Autodesk Inventor part; units mm, degrees
ref_plane "YZ Plane" through (0, 0, 0) normal (1, 0, 0) x (0, 1, 0)
ref_plane "XZ Plane" through (0, 0, 0) normal (0, 1, 0) x (-1, 0, 0)
ref_plane "XY Plane" through (0, 0, 0) normal (0, 0, 1) x (1, 0, 0)
sketch "Sketch1" plane through (0, 0, 0) normal (0, 1, 0) x (-1, 0, 0)
  line L0 (-14.4018, 8.0518) -> (14.4018, 8.0518)
  line L1 (14.4018, 8.0518) -> (14.4018, -8.0518)
  line L2 (14.4018, -8.0518) -> (-14.4018, -8.0518)
  line L3 (-14.4018, -8.0518) -> (-14.4018, 8.0518)
  line L4 (-14.4018, 8.0518) -> (14.4018, -8.0518) construction
  line L5 (14.4018, 8.0518) -> (-14.4018, -8.0518) construction
  point P0 (0, 0)
  dimension "d0" = 28.8036
  dimension "d1" = 16.1036
extrude "Extrusion1" add sketch "Sketch1" along normal blind 17.018
sketch "Sketch2" plane through (0, 17.018, 0) normal (0, 1, 0) x (1, 0, 0)
  circle A0 centre (0, 0) radius 5.9531
  dimension "d4" = 11.9062
extrude "Extrusion2" add sketch "Sketch2" along normal blind 11.811
sketch "Sketch3" plane through (0, 28.829, 0) normal (0, 1, 0) x (1, 0, 0)
  circle A0 centre (0, 0) radius 3.175
  dimension "d7" = 6.35
extrude "Extrusion3" add sketch "Sketch3" along normal blind 16.9926
fillet "Fillet1" radius 3.175 1 edges at (-3.175, 45.8216, 0)
sketch "Sketch4" plane through (0, 0, 0) normal (0, -1, 0) x (1, 0, 0)
  line L0 (-14.4018, 8.0518) -> (14.4018, 8.0518)
  line L1 (0, 8.0518) -> (3.175, 8.0518)
  line L2 (3.175, 8.0518) -> (3.175, 7.2644)
  line L3 (3.175, 7.2644) -> (0, 7.2644)
  line L4 (0, 7.2644) -> (0, 8.0518)
  line L5 (0, 8.0518) -> (-3.175, 8.0518)
  line L6 (-3.175, 8.0518) -> (-3.175, 7.2644)
  line L7 (-3.175, 7.2644) -> (0, 7.2644)
  point P0 (0, 0)
  dimension "d11" = 3.175
  dimension "d12" = 0.7874
extrude "Extrusion4" add sketch "Sketch4" along normal blind 10.795
sketch "Sketch5" plane through (0, 0, 0) normal (0, -1, 0) x (1, 0, 0)
  line L0 (14.4018, -8.0518) -> (14.4018, 8.0518)
  line L1 (14.4018, 0) -> (13.6144, 0)
  line L2 (13.6144, 0) -> (13.6144, 3.175)
  line L3 (13.6144, 3.175) -> (14.4018, 3.175)
  line L4 (14.4018, 3.175) -> (14.4018, 0)
  line L5 (13.6144, 0) -> (13.6144, -3.175)
  line L6 (13.6144, -3.175) -> (14.4018, -3.175)
  line L7 (14.4018, -3.175) -> (14.4018, 0)
  point P0 (0, 0)
  dimension "d15" = 0.7874
  dimension "d16" = 3.175
extrude "Extrusion5" add sketch "Sketch5" along normal blind 10.795
properties part number "switch toggle"
Could you check a few things on this model? Use its own coordinates, in mm. A direction names the side the tool comes from. Coordinates: 2 decimals unless noted, no trailing zeros. Order: outer loops, then holes, each group sorted by start corner. A loop starts at its lowest first (then second) coordinate and runs counter-clockwise, first axis right, second up. Notation, with made-up numbers: M 52.25,24 L 74.25,24 A21 cw 74.25,61 Z; hole C -3.5,-32 d1. An arc over 180 degrees is marked long. Use a Markdown table: item, result. Add a question column.
Q1. If I drill on L1, parallel to Y at x = -12.25, z = 4.75; L2, parallel to Y at x = -5.75, z = -1.25; L3, parallel to X at y = -5.5, z = 2.25, over which ranges is the centre line in solid material (lowest first)?
Q2. Which directions (+Z, -Z, +X, -X, +Y, -Y) give clear straight access to the entire face, cutting with the end or side of a thin tool? Please do faces 1 (the flat face through (0, -5, 7.264)), 2 (the flat face through (13.614, -5, 0)), 3 (the cylindrical face through (-0.69, 35.64, -3.1)).
Q3. I want a section at A-A on y = -6. List the corners of the cut face in (x, z) for me (3 decimals), then the cut area to 4 significant figures.
Q4. I want a section at D-D on y = 25. List the corners of the cut face in (x, z) for me, then the cut area to 3 significant figures.
Q5. I want a section at C-C on x = 0. List the corners of the cut face in (y, z) for me (3 decimals).
Q6. I'm going to push flat-ended pins straight in: pin 1 (5 mm diameter, centred on x = 1.5, z = 1.5, fed in from -Y); pin 2 (5 mm diameter, centred on x = 1, y = -7, fed in from -Z); pin 3 (7 mm diameter, centred on y = -5.5, z = -1.5, fed in from -X). Where does each tip first touch, or does it pass through?
Q7. I want a section at B-B on z = 0. List the corners of the cut face in (x, y) for me (3 decimals).
Checked values:
| question | item | result |
|---|---|---|
| 1 | L1 | 0 to 17.02 |
| 1 | L2 | 0 to 28.83 |
| 1 | L3 | 13.61 to 14.4 |
| 2 | face 1 | -Z, +X, -X, -Y |
| 2 | face 2 | +Z, -Z, -X, -Y |
| 2 | face 3 | +Y |
| 3 | outline | M -3.175,7.264 L 3.175,7.264 L 3.175,8.052 L -3.175,8.052 Z; M 13.614,-3.175 L 14.402,-3.175 L 14.402,3.175 L 13.614,3.175 Z |
| 3 | area | 10.00 mm² |
| 4 | outline | C 0,0 d11.91 |
| 4 | area | 111 mm² |
| 5 | outline | M -10.795,7.264 L 0,7.264 L 0,-8.052 L 17.018,-8.052 L 17.018,-5.953 L 28.829,-5.953 L 28.829,-3.175 L 42.647,-3.175 A3.175 ccw 42.647,3.175 L 28.829,3.175 L 28.829,5.953 L 17.018,5.953 L 17.018,8.052 L -10.795,8.052 Z |
| 6 | pin 1 | y = 0 |
| 6 | pin 2 | z = 7.26 |
| 6 | pin 3 | x = 13.61 |
| 7 | outline | M -14.402,0 L 13.614,0 L 13.614,-10.795 L 14.402,-10.795 L 14.402,17.018 L 5.953,17.018 L 5.953,28.829 L 3.175,28.829 L 3.175,42.647 A3.175 ccw -3.175,42.647 L -3.175,28.829 L -5.953,28.829 L -5.953,17.018 L -14.402,17.018 Z |
